Here's how the part is built. I have some questions about the finished solid (model axes, mm). Round coordinates to 2 decimals unless told otherwise and drop trailing zeros. Write each loop counter-clockwise with the first axis right and the second up, starting at its lowest first coordinate (ties: lowest second). Pieces come first, ordered by that corner, then holes. Notation, with made-up numbers: (-2, -10) -> (56, -10) arc R21 cw to (56, 18) -> close; hole circle Ø2 at (-33.5, -15.75). An arc over 180 degrees is marked (long way). Answer as CSV lines item,"result".
from build123d import *

# Parameters (mm, degrees)
F0_W     = 317.5
F0_H     = 292.1
F1_DEPTH = 25.4
F2_W     = 292.1
F2_H     = 12.7
F3_DEPTH = 6.35
F4_W     = 292.1
F4_H     = 12.7
F5_DEPTH = 6.35
F7_DEPTH = 6.35
F8_W     = 330.2
F8_H     = 12.7
F9_DEPTH = 6.35


with BuildPart() as f1:
    # F0 (on Top) → F1 (new body)
    with BuildSketch(Plane.XY):
        Rectangle(F0_W, F0_H)
    extrude(amount=F1_DEPTH)

    # F2 (on face) → F3 (join)
    with BuildSketch(Plane.YZ.offset(158.75)):
        with Locations((0, 12.7)):
            Rectangle(F2_W, F2_H)
    extrude(amount=F3_DEPTH)

    # F4 (on face) → F5 (join)
    with BuildSketch(Plane(origin=(-158.75, 0, 0), x_dir=(0, -1, 0), z_dir=(-1, 0, 0))):
        with Locations((0, 12.7)):
            Rectangle(F4_W, F4_H)
    extrude(amount=F5_DEPTH)

    # F6 (on face) → F7 (join)
    with BuildSketch(Plane(origin=(0, 146.05, 0), x_dir=(-1, 0, 0), z_dir=(0, 1, 0))):
        Polygon((-158.75, 19.05), (-165.1, 19.05), (-165.1, 6.35), (-158.75, 6.35), (158.75, 6.35), (165.1, 6.35), (165.1, 19.05), (158.75, 19.05), align=None)
    extrude(amount=F7_DEPTH)

    # F8 (on face) → F9 (join)
    with BuildSketch(Plane.XZ.offset(146.05)):
        with Locations((0, 12.7)):
            Rectangle(F8_W, F8_H)
    extrude(amount=F9_DEPTH)


solid = f1.part
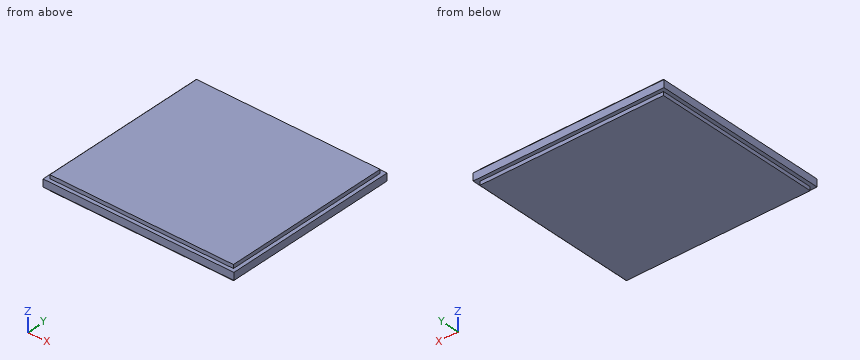
Item 1: Suppose I cut it at B-B, the plane y = 23. List the corners of the cut face in (x, z) for me, then the cut area to 3 significant figures.
Results found:
outline,"(-165.1, 6.35) -> (-158.75, 6.35) -> (-158.75, 0) -> (158.75, 0) -> (158.75, 6.35) -> (165.1, 6.35) -> (165.1, 19.05) -> (158.75, 19.05) -> (158.75, 25.4) -> (-158.75, 25.4) -> (-158.75, 19.05) -> (-165.1, 19.05) -> close"
area,"8,230 mm²"
Item 2: Suppose I cut it at A-A, the plane x = 30.5. List the corners of the cut face in (y, z) for me.
Results found:
outline,"(-152.4, 6.35) -> (-146.05, 6.35) -> (-146.05, 0) -> (146.05, 0) -> (146.05, 6.35) -> (152.4, 6.35) -> (152.4, 19.05) -> (146.05, 19.05) -> (146.05, 25.4) -> (-146.05, 25.4) -> (-146.05, 19.05) -> (-152.4, 19.05) -> close"
Item 3: I need wall thicknesses on L1, parallel to Y at x = -125, z = 5; L2, parallel to X at y = 105, z = 3.75. Which ranges of each line are inside material? Lowest first, please.
Results found:
L1,"y = -146.05 to 146.05"
L2,"x = -158.75 to 158.75"
Item 4: Will these pins go through, and if not, where does the flat tip stop? pin 1 (3 mm diameter, centred on y = 19.5, z = 21.5, fed in from -X); pin 2 (3 mm diameter, centred on x = -13.5, z = 4, fed in from +Y); pin 3 (1.9 mm diameter, centred on y = 28, z = 23, fed in from +X).
Results found:
pin 1,"stops at x = -158.75"
pin 2,"stops at y = 146.05"
pin 3,"stops at x = 158.75"
